Geometry: final body of the model. Coordinates: model frame, mm. A direction names the side the tool comes from. Coordinates: 2 decimals unless noted, no trailing zeros. Use a Markdown table: item, result. Add a question column.
Autodesk Inventor part; units mm, degrees
ref_plane "YZ Plane" through (0, 0, 0) normal (1, 0, 0) x (0, 1, 0)
ref_plane "XZ Plane" through (0, 0, 0) normal (0, 1, 0) x (-1, 0, 0)
ref_plane "XY Plane" through (0, 0, 0) normal (0, 0, 1) x (1, 0, 0)
sketch "Sketch2" plane through (0, 0, 0) normal (0, 0, 1) x (1, 0, 0)
  line L0 (-50, 78) -> (-50, 12) construction
  line L1 (-50, 12) -> (-20, 12) construction
  line L2 (-20, 12) -> (-20, 78) construction
  line L3 (-20, 78) -> (-50, 78) construction
  line L4 (-50, 78) -> (-20, 12) construction
  line L5 (-50, 12) -> (-20, 78) construction
  line L6 (-7.5, 90) -> (7.5, 90)
  line L7 (7.5, 90) -> (7.5, 0)
  line L8 (7.5, 0) -> (-7.5, 0)
  line L9 (-7.5, 0) -> (-7.5, 90)
  line L10 (-7.5, 90) -> (7.5, 0) construction
  line L11 (7.5, 90) -> (-7.5, 0) construction
  line L12 (-35, 45) -> (0, 45) construction
  line L13 (0, 45) -> (0, 0) construction
  line L14 (-7.5, 30) -> (7.5, 30)
  line L15 (7.5, 30) -> (64.1758, 30)
  circle A0 centre (0, 0) radius 115 construction
  line L16 (0, 0) -> (0, 30)
  line L17 (0, 0) -> (-99.5929, -57.5)
  line L18 (-7.5, 90) -> (-7.5, 114.7552)
  line L19 (-71.5891, -41.332) -> (-71.5891, 90)
  line L20 (-71.5891, 90) -> (-7.5, 90)
  line L21 (-22.2308, -21.4952) -> (-29.7308, -8.5048)
  line L22 (-81.6923, -38.5048) -> (-3.75, 6.4952)
  line L23 (3.75, -6.4952) -> (-74.1923, -51.4952)
  line L24 (-74.1923, -51.4952) -> (-81.6923, -38.5048)
  line L25 (-3.75, 6.4952) -> (3.75, -6.4952)
  line L26 (29.7308, -8.5048) -> (22.2308, -21.4952)
  line L27 (74.1923, -51.4952) -> (-3.75, -6.4952)
  line L28 (3.75, 6.4952) -> (81.6923, -38.5048)
  line L29 (81.6923, -38.5048) -> (74.1923, -51.4952)
  line L30 (-3.75, -6.4952) -> (3.75, 6.4952)
  point P0 (-25.9808, -15)
  point P1 (25.9808, -15)
  point P2 (-71.5891, -32.6717)
  point P3 (-25.9808, -15)
  dimension "d0" = 30
  dimension "d1" = 66
  dimension "d2" = 15
  dimension "d3" = 90
  dimension "d4" = 12.5
  dimension "d5" = 45
  dimension "d6" = 30
  dimension "d15" = 120
  dimension "d16" = 115
  dimension "d31" = 360
extrude "Extrusion1" add sketch "Sketch2" against normal blind 6 contours L9 L22 L19 L20 | L14 L16 L25 L22 L9 | L22 L25 L8 L9 | L9 L8 L17 L21 L22
hole "Hole1" at (-50, 78, 0) at (-20, 78, 0) at (-20, 12, 0) at (-50, 12, 0) direction (0, 0, -1) diameter 3.6 end through all counterbore diameter 6.5 counterbore depth 3
pattern_circular "Circular Pattern1" count 3 over 360 about axis through (0, 0, 0) along (0, 0, -1) of "Extrusion1", "Hole1"
fillet "Fillet1" radius 5 15 edges at (113.7368, 16.998, -3) (81.6923, -38.5048, -3) (-7.5, 90, -3) (-71.5891, 90, -3) (-7.5, 30, -3) (-74.1923, -51.4952, -3) (-22.2308, -21.4952, -3) (-42.1477, -106.998, -3) (29.7308, -8.5048, -3) (7.5, 78.3339, -3) (7.5, 30, -3) (22.2308, -21.4952, -3) (-29.7308, -8.5048, -3) (64.0891, -45.6621, -3) (-71.5891, -32.6717, -3)
properties part number "TestBench_Top_Motor_Support"
1) Draft query along X for faces 1 (the face through (30.21, -10.52, -3.04)), 2 (the face through (-71.589, 30, -3)), 3 (the face through (-2, -6, 0)). Return one class per face: pulls with the +X half, pulls with the -X half, needs draft (parallel to the pull), parting line crosses it, or undercut.
2) Ray query, line 1 along X through (y, z) = (12, -2.3); line 2 along Y through (x, z) = (-20, -5.15); line 3 along Y through (x, z) = (22, -3.95). Return the intervals inside material, ascending.
3) Section A-A (z = -1.55). Give the number of separate pieces and of enclosed holes in the cut face, then the cut area to 3 significant figures.
4) Set-up query: faces 4 (the face through (-48.6, 76.6, -3)), 5 (the face through (97.9, -10.43, -2.96)), 6 (the face through (61.543, 47.132, -2.958)), 7 (the face through (6.07, 31.5, -3.04)), 8 (the face through (55.41, -23.33, -2.96)). Return all of +Z, -Z, +X, -X, +Y, -Y with unobstructed straight access to the full face (end or side cutting, diameter ignored); none if empty.
5) Pin query (flat end, axial travel): pin 1 (1.5 mm diameter, centred on x = 46, y = 56, fed in from +Z); pin 2 (5 mm diameter, centred on x = 77.55, y = -21.68, fed in from +Z); pin 3 (3 mm diameter, centred on x = 1, z = -4, fed in from +Y); pin 4 (3 mm diameter, centred on x = 82.5, z = -5, fed in from -Y). Return the tip coordinate at first contact, or that it passes through.
Values follow:
| question | item | result |
|---|---|---|
| 1 | face 1 | undercut |
| 1 | face 2 | pulls with the -X half |
| 1 | face 3 | needs draft |
| 2 | line 1 | x = -71.59 to -53.25, -46.75 to -23.25, -16.75 to 17.21, 23.57 to 110.85 |
| 2 | line 2 | y = -94.21 to 10.2, 13.8 to 76.2, 79.8 to 90 |
| 2 | line 3 | y = -69.96 to 10.51, 12.13 to 69.96 |
| 3 | separate pieces | 1 |
| 3 | enclosed holes | 12 |
| 3 | area | 20,800 mm² |
| 4 | face 4 | +Z |
| 4 | face 5 | +Z, -Z, +X, -Y |
| 4 | face 6 | +Z, -Z, +X, +Y |
| 4 | face 7 | +Z, -Z, +Y |
| 4 | face 8 | +Z, -Z |
| 5 | pin 1 | stops at z = 0 |
| 5 | pin 2 | stops at z = -3 |
| 5 | pin 3 | stops at y = 30 |
| 5 | pin 4 | stops at y = -36.54 |
